Autodesk Inventor part; units mm, degrees
ref_plane "YZ Plane" through (0, 0, 0) normal (1, 0, 0) x (0, 1, 0)
ref_plane "XZ Plane" through (0, 0, 0) normal (0, 1, 0) x (-1, 0, 0)
ref_plane "XY Plane" through (0, 0, 0) normal (0, 0, 1) x (1, 0, 0)
sketch "Sketch1" plane through (0, 0, 0) normal (0, 0, 1) x (1, 0, 0)
  circle A0 centre (0, 0) radius 19.05
  circle A1 centre (0, 0) radius 9.525
  circle A2 centre (0, 0) radius 6.35
  dimension "d0" = 38.1
  dimension "d1" = 19.05
  dimension "d2" = 12.7
extrude "Extrusion1" add sketch "Sketch1" along normal mid plane 19.05 contours A0 | A1
extrude "Extrusion2" cut sketch "Sketch1" along normal mid plane 12.7 contours A0
properties part number "1.5inch_sprocket"
Can you work these out from the model? Positions are in its coordinate system, mm. A direction names the side the tool comes from. Coordinates: 2 decimals unless noted, no trailing zeros. Order: outer loops, then holes, each group sorted by start corner. A loop starts at its lowest first (then second) coordinate and runs counter-clockwise, first axis right, second up. Notation, with made-up numbers: (-17, 12) - (21, 12) arc R23 ccw to (21, 41) - close; hole circle Ø6 at (78.25, 28.25). An arc over 180 degrees is marked (long way). Answer in a Markdown table with one row per item.
1. Suppose I cut it at A-A (x = 0). Please give me the cut outline in (y, z) (3 decimals).
Reply:
| item | result |
|---|---|
| outline | (-19.05, -9.525) - (-6.35, -9.525) - (-6.35, 9.525) - (-19.05, 9.525) - (-19.05, 6.35) - (-9.525, 6.35) - (-9.525, -6.35) - (-19.05, -6.35) - close; (6.35, -9.525) - (19.05, -9.525) - (19.05, -6.35) - (9.525, -6.35) - (9.525, 6.35) - (19.05, 6.35) - (19.05, 9.525) - (6.35, 9.525) - close |
2. Suppose I cut it at D-D (x = 13). Please give me the cut outline in (y, z) (3 decimals).
Reply:
| item | result |
|---|---|
| outline | (-13.925, -9.525) - (13.925, -9.525) - (13.925, -6.35) - (-13.925, -6.35) - close; (-13.925, 6.35) - (13.925, 6.35) - (13.925, 9.525) - (-13.925, 9.525) - close |
3. For faces 4 (the flat face through (-5, 5, 9.525)), 5 (the cylindrical face through (-7.559, -5.796, 0.089)), which set-ups out of +Z, -Z, +X, -X, +Y, -Y let a thin tool reach every point of the face, with its end or its side?
Reply:
| item | result |
|---|---|
| face 4 | +Z, +X, -X, +Y, -Y |
| face 5 | none |
4. If we mould it in two halves opening along Y, with no side actions, what happens to faces 1 (the cylindrical face through (-1.38, 6.2, -0.13)), 2 (the cylindrical face through (-15.12, -11.59, 7.96)), 3 (the flat face through (-5, 5, -9.525))? For each: pulls with the +Y half, pulls with the -Y half, needs draft (parallel to the pull), parting line crosses it, or undercut.
Reply:
| item | result |
|---|---|
| face 1 | undercut |
| face 2 | parting line crosses it |
| face 3 | needs draft |
5. Suppose I cut it at C-C (z = 1.5). Please give me the cut outline in (x, y) (3 decimals), and give its area (3 significant figures).
Reply:
| item | result |
|---|---|
| outline | circle Ø19.05 at (0, 0); hole circle Ø12.7 at (0, 0) |
| area | 158 mm^2 |
6. For pin 1 (6 mm diameter, centred on x = 11.5, z = 7.5, fed in from +Y); pin 2 (4 mm diameter, centred on x = -1.5, z = 4.5, fed in from -Y); pin 3 (5 mm diameter, centred on y = 8.5, z = -6, fed in from -X), each with a flat end and sliding along its axis, tell me the tip position at first contact or that it passes through.
Reply:
| item | result |
|---|---|
| pin 1 | stops at y = 17.05 |
| pin 2 | stops at y = -19.04 |
| pin 3 | stops at x = -18.07 |
7. If I drill on line 1 along Z through (x, y) = (3, 12) (3 decimals); line 2 along Y through (x, z) = (0, -7.5), over which ranges is the centre line in solid material (lowest first)?
Reply:
| item | result |
|---|---|
| line 1 | z = -9.525 to -6.35, 6.35 to 9.525 |
| line 2 | y = -19.05 to -6.35, 6.35 to 19.05 |
